Geometry: final body of the model. Coordinates: model frame, mm. A direction names the side the tool comes from. Coordinates: 2 decimals unless noted, no trailing zeros. Write each loop counter-clockwise with the first axis right and the second up, starting at its lowest first coordinate (ties: lowest second). Pieces come first, ordered by that corner, then holes.
from build123d import *

# Parameters (mm, degrees)
CROQUIS1_R                  = 1.5
SALIENTE_EXTRUIR1_DEPTH     = 5
SALIENTE_EXTRUIR2_DEPTH     = 4
REVOLUCI_N1_ANGLE           = 70
REVOLUCI_N1_OTHER_WAY_ANGLE = 70
REVOLUCI_N2_ANGLE           = 70
REVOLUCI_N2_OTHER_WAY_ANGLE = 70
CHAFL_N1_SIZE               = 1.5


with BuildPart() as part:
    # Croquis1 → Saliente-Extruir1 (new body)
    with BuildSketch(Plane(origin=(0, 0, 0), x_dir=(1, 0, 0), z_dir=(0, 1, 0))):
        with BuildLine():
            Line((-12, 4), (12, 4))
            ThreePointArc((12, 4), (16, 0), (12, -4))
            Line((12, -4), (-12, -4))
            ThreePointArc((-12, -4), (-16, 0), (-12, 4))
        make_face()
        with Locations(Location((12, 0, 0), (0, 0, 270))):
            Circle(CROQUIS1_R, mode=Mode.SUBTRACT)
        with Locations(Location((-12, 0, 0), (0, 0, 270))):
            Circle(CROQUIS1_R, mode=Mode.SUBTRACT)
    extrude(amount=SALIENTE_EXTRUIR1_DEPTH)

    # Croquis2 → Saliente-Extruir2 (add)
    with BuildSketch(Plane(origin=(0, 5, 0), x_dir=(1, 0, 0), z_dir=(0, 1, 0))):
        with BuildLine():
            Line((-3.47706773, -4), (-0.9, -4))
            ThreePointArc((-0.9, -4), (-4.1, 0), (-0.9, 4))
            Line((-0.9, 4), (-3.47706773, 4))
            ThreePointArc((-3.47706773, 4), (-5.3, 0), (-3.47706773, -4))
        make_face()
        with BuildLine():
            Line((0.9, -4), (3.47706773, -4))
            ThreePointArc((3.47706773, -4), (5.3, 0), (3.47706773, 4))
            Line((3.47706773, 4), (0.9, 4))
            ThreePointArc((0.9, 4), (4.1, 0), (0.9, -4))
        make_face()
    extrude(amount=SALIENTE_EXTRUIR2_DEPTH)

    # Croquis4 → Revolución1 (revolve)
    with BuildSketch(Plane.XY):
        with BuildLine():
            Line((4.1, 9), (5.3, 9))
            ThreePointArc((5.3, 9), (5.219481091, 9.920335342), (4.98037089, 10.81270676))
            Line((4.98037089, 10.81270676), (3.852739745, 10.402282588))
            ThreePointArc((3.852739745, 10.402282588), (4.037711787, 9.711957528), (4.1, 9))
        make_face()
    revolve(axis=Axis((0, 9, 0), (0, 1, 0)), revolution_arc=REVOLUCI_N1_ANGLE)

    # Croquis4 → Revolución1 other way (revolve)
    with BuildSketch(Plane.XY):
        with BuildLine():
            Line((4.1, 9), (5.3, 9))
            ThreePointArc((5.3, 9), (5.219481091, 9.920335342), (4.98037089, 10.81270676))
            Line((4.98037089, 10.81270676), (3.852739745, 10.402282588))
            ThreePointArc((3.852739745, 10.402282588), (4.037711787, 9.711957528), (4.1, 9))
        make_face()
    revolve(axis=Axis((0, 9, 0), (0, -1, 0)), revolution_arc=REVOLUCI_N1_OTHER_WAY_ANGLE)

    # Croquis5 → Revolución2 (revolve)
    with BuildSketch(Plane.XY):
        with BuildLine():
            Line((-5.3, 9), (-4.1, 9))
            ThreePointArc((-4.1, 9), (-4.037711787, 9.711957528), (-3.852739745, 10.402282588))
            Line((-3.852739745, 10.402282588), (-4.98037089, 10.81270676))
            ThreePointArc((-4.98037089, 10.81270676), (-5.219481091, 9.920335342), (-5.3, 9))
        make_face()
    revolve(axis=Axis((0, 9, 0), (0, 1, 0)), revolution_arc=REVOLUCI_N2_ANGLE)

    # Croquis5 → Revolución2 other way (revolve)
    with BuildSketch(Plane.XY):
        with BuildLine():
            Line((-5.3, 9), (-4.1, 9))
            ThreePointArc((-4.1, 9), (-4.037711787, 9.711957528), (-3.852739745, 10.402282588))
            Line((-3.852739745, 10.402282588), (-4.98037089, 10.81270676))
            ThreePointArc((-4.98037089, 10.81270676), (-5.219481091, 9.920335342), (-5.3, 9))
        make_face()
    revolve(axis=Axis((0, 9, 0), (0, -1, 0)), revolution_arc=REVOLUCI_N2_OTHER_WAY_ANGLE)

    # Chaflán1
    chafl_n1_edges = [part.edges().sort_by_distance(p)[0] for p in [
        (-5.3, 5, 0),
        (5.3, 5, 0),
    ]]
    chamfer(chafl_n1_edges, length=CHAFL_N1_SIZE)


solid = part.part
Item 1: Section A-A, the plane y = 8.5. Output: boundary loops of the cut face in (x, z), plus the area to 3 significant figures.
Derived:
outline: (-3.48, -4) - (-0.9, -4) arc R4.1 cw to (-0.9, 4) - (-3.48, 4) arc R5.3 ccw to start; (0.9, -4) - (3.48, -4) arc R5.3 ccw to (3.48, 4) - (0.9, 4) arc R4.1 cw to start
area: 23.3 mm2
Item 2: Section C-C, the plane y = 4.5. Output: boundary loops of the cut face in (x, z).
Derived:
outline: (-12, -4) - (12, -4) arc R4 ccw to (12, 4) - (-12, 4) arc R4 ccw to start; hole circle Ø3 at (-12, 0); hole circle Ø3 at (12, 0)
Item 3: Pin query (flat end, axial travel): pin 1 (5 mm diameter, centred on x = 12.5, y = 1.5, fed in from -Z); pin 2 (1 mm diameter, centred on x = -8.5, z = -1, fed in from +Y); pin 3 (4.5 mm diameter, centred on x = -1.5, y = 3, fed in from +Z). Return the tip coordinate at first contact, or that it passes through.
Derived:
pin 1: stops at z = -4
pin 2: stops at y = 5
pin 3: stops at z = 4
Item 4: Material intervals for probe 1 along X at (y, z) = (1.95, 0); probe 2 along X at (y, z) = (2, -1); probe 3 along Y at (x, z) = (1.5, 1.5), sorted ascending.
Derived:
probe 1: x = -16 to -13.5, -10.5 to 10.5, 13.5 to 16
probe 2: x = -15.87 to -13.12, -10.88 to 10.88, 13.12 to 15.87
probe 3: y = 0 to 5
Item 5: Set-up query: faces 4 (the flat face through (-2.2, 9, 4.4)), 5 (the cylindrical face through (5.3, 7.7, 0.1)), 6 (the conical face through (4.032, 10.468, -0.069)), 7 (the flat face through (1.56, 9.92, -4.29)), 8 (the cylindrical face through (-4.1, 7, 0.1)). Return all of +Z, -Z, +X, -X, +Y, -Y with unobstructed straight access to the full face (end or side cutting, diameter ignored); none if empty.
Derived:
face 4: +Z, +X, -X, -Y
face 5: +X, +Y
face 6: +Y
face 7: -Z, +Y
face 8: none
Item 6: Pull-direction query (Y, two-part tool) for faces 1 (the cylindrical face through (4.1, 7, -0.1)), 2 (the cylindrical face through (16, 2, 0)), 3 (the flat face through (2.3, 9, -4.4)); classes: released by +Y, released by -Y, zero draft, split by the parting line, or undercut.
Derived:
face 1: undercut
face 2: zero draft
face 3: released by -Y
Item 7: Section D-D, the plane x = -8. Output: boundary loops of the cut face in (y, z), plus the area to 3 significant figures.
Derived:
outline: (0, -4) - (5, -4) - (5, 4) - (0, 4) - close
area: 40.0 mm2
Item 8: Section B-B, the plane z = 0. Output: boundary loops of the cut face in (x, y).
Derived:
outline: (-16, 0) - (-13.5, 0) - (-13.5, 5) - (-16, 5) - close; (-10.5, 0) - (10.5, 0) - (10.5, 5) - (6.8, 5) - (5.3, 6.5) - (5.3, 9) arc R5.3 ccw to (4.98, 10.81) - (3.85, 10.4) arc R4.1 cw to (4.1, 9) - (4.1, 5) - (-4.1, 5) - (-4.1, 9) arc R4.1 cw to (-3.85, 10.4) - (-4.98, 10.81) arc R5.3 ccw to (-5.3, 9) - (-5.3, 6.5) - (-6.8, 5) - (-10.5, 5) - close; (13.5, 0) - (16, 0) - (16, 5) - (13.5, 5) - close
